Read the model definition and answer for the solid it produces. Units are mm, in the model's axes. Coordinates: 2 decimals unless noted, no trailing zeros. Loops run counter-clockwise (first coordinate to the right, second up) from the corner with the lowest first, then second, coordinate; pieces in that order, holes last.
Autodesk Inventor part; units mm, degrees
ref_plane "YZ Plane" through (0, 0, 0) normal (1, 0, 0) x (0, 1, 0)
ref_plane "XZ Plane" through (0, 0, 0) normal (0, 1, 0) x (-1, 0, 0)
ref_plane "XY Plane" through (0, 0, 0) normal (0, 0, 1) x (1, 0, 0)
sketch "Sketch1" plane through (0, 0, 0) normal (0, 1, 0) x (-1, 0, 0)
  line L0 (55, 312.5) -> (-55, 312.5)
  line L1 (-55, 312.5) -> (-55, -312.5)
  line L2 (-55, -312.5) -> (55, -312.5)
  line L3 (55, -312.5) -> (55, 312.5)
  line L4 (55, 312.5) -> (-55, -312.5) construction
  line L5 (-55, 312.5) -> (55, -312.5) construction
  line L6 (0, 0) -> (-55, 0)
  line L7 (-55, 0) -> (-25, 0)
  line L8 (-25, 0) -> (-25, -78)
  line L9 (-25, -78) -> (-25, 78)
  line L10 (-25, 78) -> (-55, 78)
  line L11 (-25, -78) -> (-55, -78)
  dimension "d0" = 110
  dimension "d1" = 625
  dimension "d2" = 30
  dimension "d3" = 78
  dimension "d4" = 156
extrude "Extrusion1" add sketch "Sketch1" along normal blind 3 contours L3 L2 L1 L11 L8 L9 L10 L0
properties part number "border2"
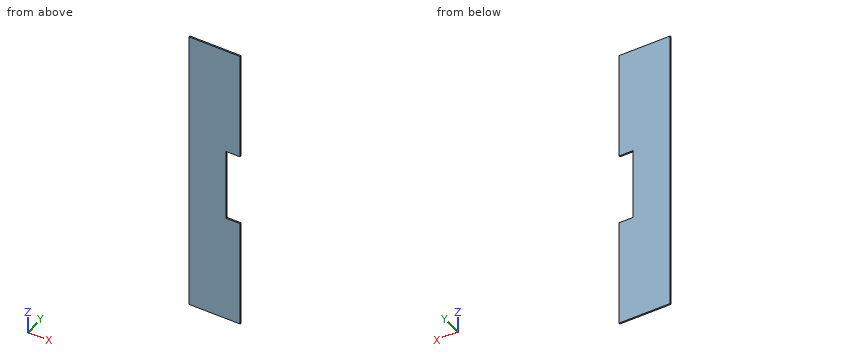
Item 1: Given pin 1 (1.5 mm diameter, centred on y = 2, z = -2.5, fed in from +X), flat-ended and moving along its own axis, determine where the tip first touches the part or whether it passes through.
Numbers:
pin 1: stops at x = 25
Item 2: Find the intervals of material crossed by line 1 along Z through (x, y) = (42, 2.95); line 2 along X through (y, z) = (0.6, 77), in increasing order.
Numbers:
line 1: z = -312.5 to -78, 78 to 312.5
line 2: x = -55 to 25
Item 3: A cutting plane is placed at B-B on y = 0.9. Determine the outline of the cut face in (x, z), then the cut area to 3 significant figures.
Numbers:
outline: (-55, -312.5) - (55, -312.5) - (55, -78) - (25, -78) - (25, 78) - (55, 78) - (55, 312.5) - (-55, 312.5) - close
area: 64,100 mm2
Item 4: A cutting plane is placed at A-A on x = 41. Determine the outline of the cut face in (y, z), then the cut area to 3 significant figures.
Numbers:
outline: (0, -312.5) - (3, -312.5) - (3, -78) - (0, -78) - close; (0, 78) - (3, 78) - (3, 312.5) - (0, 312.5) - close
area: 1,410 mm2
